```python
from build123d import *

# Parameters (mm, degrees)
SKETCH_1_W                   = 45
SKETCH_1_H                   = 45
EXTRUDE_1_DEPTH              = 5
HOLE_WIZARD_M3_3_D           = 2.5
HOLE_WIZARD_M3_3_CSINK_D     = 3.05
HOLE_WIZARD_M3_3_CSINK_ANGLE = 90


with BuildPart() as part:
    # 草图1 → 凸台-拉伸1 (new body)
    with BuildSketch(Plane.XY):
        with Locations((22.5, 22.5)):
            Rectangle(SKETCH_1_W, SKETCH_1_H)
    extrude(amount=EXTRUDE_1_DEPTH)

    # M3 螺纹孔3 (through all)
    with Locations(Plane.XY.offset(5)):
        with Locations((12.5, 35), (32.5, 35), (32.5, 15), (12.5, 15)):
            CounterSinkHole(HOLE_WIZARD_M3_3_D / 2, HOLE_WIZARD_M3_3_CSINK_D / 2, counter_sink_angle=HOLE_WIZARD_M3_3_CSINK_ANGLE)


solid = part.part
```
Read the model definition and answer for the solid it produces. Units are mm, in the model's axes. Give positions to 0.01 mm unless a question says otherwise; leave off trailing zeros. Write each loop counter-clockwise with the first axis right and the second up, starting at its lowest first coordinate (ties: lowest second). Pieces come first, ordered by that corner, then holes. Notation, with made-up numbers: (14.25, -12) - (28.25, -12) arc R9 cw to (28.25, 3) - close; hole circle Ø11 at (31.25, 78.25). An arc over 180 degrees is marked (long way). Write item = value, one per line. Start each with the question number.
Item 1: The mould has two halves that part along X. Classify faces 1 (the flat face through (45, 22, 2)), 2 (the flat face through (22, 23, 0)), 3 (the cylindrical face through (13.421, 15.845, 2.329)): +X half, -X half, draft (parallel to the pull), parting line (faces both ways), or undercut.
Item 2: Find section A-A (x = 32.5). Give the vertices of the cut face in (y, z) (3 decimals).
Item 3: This flat-tipped pin is pushed along its axis until it touches: P1, Ø3, axis at x = 12.5, y = 15, coming from the +Z side (3 decimals). Where does it stop, or does it pass through?
Item 4: Find section B-B (y = 15). Give the vertices of the cut face in (x, z) (3 decimals).
Item 5: Find the intervals of material crossed by probe 1 along X at (y, z) = (35, 3); probe 2 along Y at (x, z) = (12.5, 3.2); probe 3 along X at (y, z) = (16, 2.65), in increasing order. Write a range as [from, to].
Response:
q1.face_1 = +X half
q1.face_2 = draft
q1.face_3 = undercut
q2.outline = (0, 0) - (13.75, 0) - (13.75, 4.725) - (13.475, 5) - (0, 5) - close; (16.25, 0) - (33.75, 0) - (33.75, 4.725) - (33.475, 5) - (16.525, 5) - (16.25, 4.725) - close; (36.25, 0) - (45, 0) - (45, 5) - (36.525, 5) - (36.25, 4.725) - close
q3.P1 = 4.975
q4.outline = (0, 0) - (11.25, 0) - (11.25, 4.725) - (10.975, 5) - (0, 5) - close; (13.75, 0) - (31.25, 0) - (31.25, 4.725) - (30.975, 5) - (14.025, 5) - (13.75, 4.725) - close; (33.75, 0) - (45, 0) - (45, 5) - (34.025, 5) - (33.75, 4.725) - close
q5.probe_1 = [0, 11.25], [13.75, 31.25], [33.75, 45]
q5.probe_2 = [0, 13.75], [16.25, 33.75], [36.25, 45]
q5.probe_3 = [0, 11.75], [13.25, 31.75], [33.25, 45]
